```python
from build123d import *

# Parameters (mm, degrees)
SKETCH1_W                       = 108
SKETCH1_H                       = 86
BOSS_EXTRUDE1_DEPTH             = 2
SKETCH2_W                       = 104
SKETCH2_H                       = 82
SKETCH2_W_2                     = 101
SKETCH2_H_2                     = 79
BOSS_EXTRUDE2_DEPTH             = 3
BOSS_EXTRUDE4_REACH             = 138.591
SKETCH5_W                       = 10
SKETCH5_H                       = 10
BOSS_EXTRUDE4_DIRECTION_2_REACH = 138.591
BOSS_EXTRUDE5_REACH             = 139.026
SKETCH6_W                       = 10
SKETCH6_H                       = 10
BOSS_EXTRUDE5_DIRECTION_2_REACH = 139.026
SKETCH11_W                      = 0.1
SKETCH11_H                      = 10
SKETCH11_W_2                    = 0.2
CUT_EXTRUDE2_DEPTH              = 10
CHAMFER1_SIZE                   = 0.5
CHAMFER2_SIZE                   = 0.5
CUT_EXTRUDE3_REACH              = 140.578
SKETCH12_R                      = 1.375
CUT_EXTRUDE5_DEPTH              = 3
CUT_EXTRUDE6_REACH              = 140.501
SKETCH14_R                      = 1.925
CUT_EXTRUDE7_REACH              = 140.423
SKETCH15_R                      = 1.925


with BuildPart() as part:
    # Sketch1 → Boss-Extrude1 (new body)
    with BuildSketch(Plane(origin=(0, 0, 0), x_dir=(1, 0, 0), z_dir=(0, 1, 0))):
        with Locations((54, 43)):
            Rectangle(SKETCH1_W, SKETCH1_H)
    extrude(amount=BOSS_EXTRUDE1_DEPTH)

    # Sketch2 → Boss-Extrude2 (add)
    with BuildSketch(Plane(origin=(0, 2, 0), x_dir=(1, 0, 0), z_dir=(0, 1, 0))):
        with Locations((54, 43)):
            Rectangle(SKETCH2_W, SKETCH2_H)
        with Locations((54, 43)):
            Rectangle(SKETCH2_W_2, SKETCH2_H_2, mode=Mode.SUBTRACT)
    extrude(amount=BOSS_EXTRUDE2_DEPTH)

    # Boss-Extrude4: up to this face of the body (flat: up to its plane)
    boss_extrude4_end = Plane(part.part.faces().sort_by_distance((0, 1, -43))[0])
    # Sketch5 → Boss-Extrude4 (add, up to the picked face)
    with BuildSketch(Plane.ZY.offset(-2), mode=Mode.PRIVATE) as boss_extrude4_sk1:
        with Locations((-43, 7)):
            Rectangle(SKETCH5_W, SKETCH5_H)
    boss_extrude4_tool1 = split(extrude(boss_extrude4_sk1.sketch, amount=BOSS_EXTRUDE4_REACH, mode=Mode.PRIVATE), bisect_by=boss_extrude4_end, keep=Keep.BOTH, mode=Mode.PRIVATE)
    add(boss_extrude4_tool1.solids().sort_by(Axis((2, 7, -43), (-1, 0, 0)))[0])

    # Boss-Extrude4 direction 2: up to this face of the body (flat: up to its plane)
    boss_extrude4_direction_2_end = Plane(part.part.faces().sort_by_distance((3.5, 3.5, -43))[0])
    # Sketch5 → Boss-Extrude4 direction 2 (add, up to the picked face)
    with BuildSketch(Plane.ZY.offset(-2), mode=Mode.PRIVATE) as boss_extrude4_direction_2_sk1:
        with Locations((-43, 7)):
            Rectangle(SKETCH5_W, SKETCH5_H)
    boss_extrude4_direction_2_tool1 = split(extrude(boss_extrude4_direction_2_sk1.sketch, amount=-BOSS_EXTRUDE4_DIRECTION_2_REACH, mode=Mode.PRIVATE), bisect_by=boss_extrude4_direction_2_end, keep=Keep.BOTH, mode=Mode.PRIVATE)
    add(boss_extrude4_direction_2_tool1.solids().sort_by(Axis((2, 7, -43), (1, 0, 0)))[0])

    # Boss-Extrude5: up to this face of the body (flat: up to its plane)
    boss_extrude5_end = Plane(part.part.faces().sort_by_distance((108, 1, -43))[0])
    # Sketch6 → Boss-Extrude5 (add, up to the picked face)
    with BuildSketch(Plane(origin=(106, 0, 0), x_dir=(0, 0, -1), z_dir=(1, 0, 0)), mode=Mode.PRIVATE) as boss_extrude5_sk1:
        with Locations((43, 7)):
            Rectangle(SKETCH6_W, SKETCH6_H)
    boss_extrude5_tool1 = split(extrude(boss_extrude5_sk1.sketch, amount=BOSS_EXTRUDE5_REACH, mode=Mode.PRIVATE), bisect_by=boss_extrude5_end, keep=Keep.BOTH, mode=Mode.PRIVATE)
    add(boss_extrude5_tool1.solids().sort_by(Axis((106, 7, -43), (1, 0, 0)))[0])

    # Boss-Extrude5 direction 2: up to this face of the body (flat: up to its plane)
    boss_extrude5_direction_2_end = Plane(part.part.faces().sort_by_distance((104.5, 3.5, -43))[0])
    # Sketch6 → Boss-Extrude5 direction 2 (add, up to the picked face)
    with BuildSketch(Plane(origin=(106, 0, 0), x_dir=(0, 0, -1), z_dir=(1, 0, 0)), mode=Mode.PRIVATE) as boss_extrude5_direction_2_sk1:
        with Locations((43, 7)):
            Rectangle(SKETCH6_W, SKETCH6_H)
    boss_extrude5_direction_2_tool1 = split(extrude(boss_extrude5_direction_2_sk1.sketch, amount=-BOSS_EXTRUDE5_DIRECTION_2_REACH, mode=Mode.PRIVATE), bisect_by=boss_extrude5_direction_2_end, keep=Keep.BOTH, mode=Mode.PRIVATE)
    add(boss_extrude5_direction_2_tool1.solids().sort_by(Axis((106, 7, -43), (-1, 0, 0)))[0])

    # Sketch11 → Cut-Extrude2 (cut)
    with BuildSketch(Plane(origin=(0, 12, 0), x_dir=(1, 0, 0), z_dir=(0, 1, 0))):
        with Locations((0.05, 43)):
            Rectangle(SKETCH11_W, SKETCH11_H)
        with Locations((107.9, 43)):
            Rectangle(SKETCH11_W_2, SKETCH11_H)
    extrude(amount=-CUT_EXTRUDE2_DEPTH, mode=Mode.SUBTRACT)

    # Chamfer1
    chamfer1_edges = [part.edges().sort_by_distance(p)[0] for p in [
        (54, 5, -84),
        (2, 5, -66),
        (54, 5, -2),
        (106, 5, -20),
        (2, 5, -20),
        (106, 5, -66),
    ]]
    chamfer(chamfer1_edges, length=CHAMFER1_SIZE)

    # Chamfer2
    chamfer2_edges = [part.edges().sort_by_distance(p)[0] for p in [
        (106.15, 12, -38),
        (106.15, 12, -48),
        (1.8, 12, -48),
        (1.8, 12, -38),
        (0.1, 12, -43),
        (107.8, 12, -43),
    ]]
    chamfer(chamfer2_edges, length=CHAMFER2_SIZE)

    # Sketch12 → Cut-Extrude3 (cut, up to next)
    with BuildSketch(Plane.XZ, mode=Mode.PRIVATE) as cut_extrude3_sk1:
        with Locations(Location((100, -78.425, 0), (0, 0, 270))):
            Circle(SKETCH12_R)
    cut_extrude3_tool1 = extrude(cut_extrude3_sk1.sketch, amount=-CUT_EXTRUDE3_REACH, mode=Mode.PRIVATE) & part.part
    # Sketch12 → Cut-Extrude3 (cut, up to next)
    with BuildSketch(Plane.XZ, mode=Mode.PRIVATE) as cut_extrude3_sk2:
        with Locations(Location((8, -78.425, 0), (0, 0, 270))):
            Circle(SKETCH12_R)
    cut_extrude3_tool2 = extrude(cut_extrude3_sk2.sketch, amount=-CUT_EXTRUDE3_REACH, mode=Mode.PRIVATE) & part.part
    # Sketch12 → Cut-Extrude3 (cut, up to next)
    with BuildSketch(Plane.XZ, mode=Mode.PRIVATE) as cut_extrude3_sk3:
        with Locations(Location((8, -20.425, 0), (0, 0, 270))):
            Circle(SKETCH12_R)
    cut_extrude3_tool3 = extrude(cut_extrude3_sk3.sketch, amount=-CUT_EXTRUDE3_REACH, mode=Mode.PRIVATE) & part.part
    # Sketch12 → Cut-Extrude3 (cut, up to next)
    with BuildSketch(Plane.XZ, mode=Mode.PRIVATE) as cut_extrude3_sk4:
        with Locations(Location((100, -20.425, 0), (0, 0, 270))):
            Circle(SKETCH12_R)
    cut_extrude3_tool4 = extrude(cut_extrude3_sk4.sketch, amount=-CUT_EXTRUDE3_REACH, mode=Mode.PRIVATE) & part.part
    add(cut_extrude3_tool1.solids().sort_by_distance((100, 0, -78.425))[0], mode=Mode.SUBTRACT)
    add(cut_extrude3_tool2.solids().sort_by_distance((8, 0, -78.425))[0], mode=Mode.SUBTRACT)
    add(cut_extrude3_tool3.solids().sort_by_distance((8, 0, -20.425))[0], mode=Mode.SUBTRACT)
    add(cut_extrude3_tool4.solids().sort_by_distance((100, 0, -20.425))[0], mode=Mode.SUBTRACT)

    # Sketch13 → Cut-Extrude5 (cut)
    with BuildSketch(Plane(origin=(0, 5, 0), x_dir=(1, 0, 0), z_dir=(0, 1, 0))):
        Polygon((3.35, 38), (3.35, 3.35), (104.65, 3.35), (104.65, 38), (104.5, 38), (104.5, 3.5), (3.5, 3.5), (3.5, 38), align=None)
    extrude(amount=-CUT_EXTRUDE5_DEPTH, mode=Mode.SUBTRACT)

    # Sketch14 → Cut-Extrude6 (cut, up to next)
    with BuildSketch(Plane.ZY.offset(-0.1), mode=Mode.PRIVATE) as cut_extrude6_sk1:
        with Locations((-43, 7.15)):
            Circle(SKETCH14_R)
    cut_extrude6_tool1 = extrude(cut_extrude6_sk1.sketch, amount=-CUT_EXTRUDE6_REACH, mode=Mode.PRIVATE) & part.part
    add(cut_extrude6_tool1.solids().sort_by_distance((0.1, 7.15, -43))[0], mode=Mode.SUBTRACT)

    # Sketch15 → Cut-Extrude7 (cut, up to next)
    with BuildSketch(Plane(origin=(107.8, 0, 0), x_dir=(0, 0, -1), z_dir=(1, 0, 0)), mode=Mode.PRIVATE) as cut_extrude7_sk1:
        with Locations(Location((43, 7.15, 0), (0, 0, 180))):
            Circle(SKETCH15_R)
    cut_extrude7_tool1 = extrude(cut_extrude7_sk1.sketch, amount=-CUT_EXTRUDE7_REACH, mode=Mode.PRIVATE) & part.part
    add(cut_extrude7_tool1.solids().sort_by_distance((107.8, 7.15, -43))[0], mode=Mode.SUBTRACT)


solid = part.part
```
Geometry: final body of the model. Coordinates: model frame, mm. A direction names the side the tool comes from. Coordinates: 2 decimals unless noted, no trailing zeros. Write each loop counter-clockwise with the first axis right and the second up, starting at its lowest first coordinate (ties: lowest second). Pieces come first, ordered by that corner, then holes. Notation, with made-up numbers: M 63,76 L 75,76 A21 cw 75,81 Z; hole C 60,49.25 d3. An arc over 180 degrees is marked long. Answer as CSV lines item,"result". Start each with the question number.
Q1. Pin query (flat end, axial travel): P1, Ø3.5, axis at x = 1.5, y = 5, coming from the +Z side; P2, Ø1, axis at x = 77.5, z = -49, coming from the +Y side; P3, Ø2.5, axis at x = 8, z = -78.425, coming from the -Y side; P4, Ø0.8, axis at y = 3.5, z = -23, coming from the +X side. Return the tip coordinate at first contact, or that it passes through.
Q2. Cut plane D-D on z = -69.5. Return the cut outline in (x, y), then the cut area to 3 significant figures.
Q3. Cut plane A-A on z = -43. Return the cut outline in (x, y) (3 decimals), then the cut area to 3 significant figures.
Q4. Cut plane C-C on y = 7.15. Return the cut outline in (x, z) (3 decimals).
Q5. Reachability of faces 1 (the flat face through (106, 3, -66)), 2 (the flat face through (53, 3, -84)), 3 (the flat face through (3.5, 4.7, -55)) from +Z, -Z, +X, -X, +Y, -Y: full face, straight path, thin tool, end or side. Return the list, or none.
Q6. Line query: line 1 (Z direction, x = 100, y = 1.4); line 2 (Z direction, x = 32, y = 3); line 3 (Y direction, x = 1.7, z = -43) (3 decimals). Output: solid intervals per line, ascending. Write a range as from..to.
Q7. Mould query, pull axis X, two halves, no side actions, for faces 4 (the flat face through (53, 3, -82.5)), 5 (the flat face through (2, 3, -20)), 6 (the flat face through (106, 3, -20)), 7 (the flat face through (1.7, 2, -36.8)). Classes: released by +X, released by -X, zero draft, split by the parting line, or undercut.
Q8. Cut plane B-B on x = 8. Return the cut outline in (y, z).
Findings below:
1,P1,"stops at z = -2"
1,P2,"stops at y = 2"
1,P3,"passes through"
1,P4,"stops at x = 106"
2,outline,"M 0,0 L 108,0 L 108,2 L 106,2 L 106,4.5 L 105.5,5 L 104.5,5 L 104.5,2 L 3.5,2 L 3.5,5 L 2.5,5 L 2,4.5 L 2,2 L 0,2 Z"
2,area,"225 mm2"
3,outline,"M 0,0 L 108,0 L 108,2 L 107.8,2 L 107.8,5.225 L 104.5,5.225 L 104.5,2 L 3.5,2 L 3.5,5.225 L 0.1,5.225 L 0.1,2 L 0,2 Z; M 0.1,9.075 L 3.5,9.075 L 3.5,12 L 0.6,12 L 0.1,11.5 Z; M 104.5,9.075 L 107.8,9.075 L 107.8,11.5 L 107.3,12 L 104.5,12 Z"
3,area,"257 mm2"
4,outline,"M 0.1,-48 L 3.5,-48 L 3.5,-44.925 L 0.1,-44.925 Z; M 0.1,-41.075 L 3.5,-41.075 L 3.5,-38 L 0.1,-38 Z; M 104.5,-48 L 107.8,-48 L 107.8,-44.925 L 104.5,-44.925 Z; M 104.5,-41.075 L 107.8,-41.075 L 107.8,-38 L 104.5,-38 Z"
5,face 1,"-Z, +X, +Y"
5,face 2,"-Z, +X, -X, +Y"
5,face 3,"+Y"
6,line 1,"z = -86..-79.8, -77.05..-21.8, -19.05..0"
6,line 2,"z = -84..-82.5, -3.35..-2"
6,line 3,"y = 0..5.225, 9.075..12"
7,face 4,"undercut"
7,face 5,"released by -X"
7,face 6,"released by +X"
7,face 7,"zero draft"
8,outline,"M 0,-86 L 2,-86 L 2,-84 L 4.5,-84 L 5,-83.5 L 5,-82.5 L 2,-82.5 L 2,-79.8 L 0,-79.8 Z; M 0,-77.05 L 2,-77.05 L 2,-21.8 L 0,-21.8 Z; M 0,-19.05 L 2,-19.05 L 2,-3.35 L 5,-3.35 L 5,-2.5 L 4.5,-2 L 2,-2 L 2,0 L 0,0 Z"
